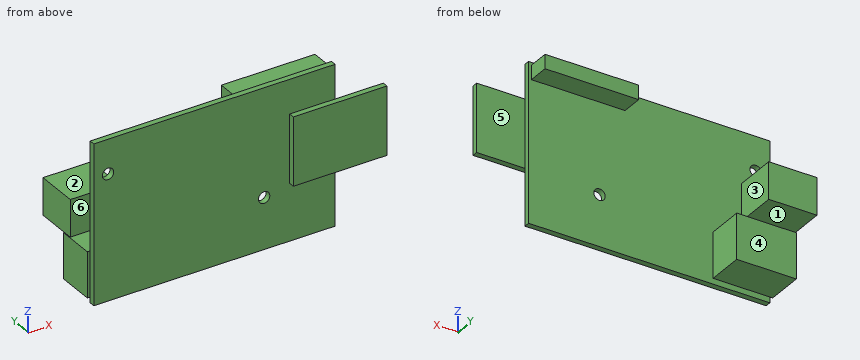
from build123d import *

# Parameters (mm, degrees)
SKETCH1_W           = 85
SKETCH1_H           = 56
BOSS_EXTRUDE1_DEPTH = 2
SKETCH2_W           = 21
SKETCH2_H           = 16
BOSS_EXTRUDE2_DEPTH = 13
SKETCH3_W           = 17
SKETCH3_H           = 13
BOSS_EXTRUDE3_DEPTH = 15
SKETCH4_W           = 33
SKETCH4_H           = 24
BOSS_EXTRUDE4_DEPTH = 2
CUT_EXTRUDE1_REACH  = 6
SKETCH5_R           = 2
SKETCH6_W           = 33
SKETCH6_H           = 5
BOSS_EXTRUDE5_DEPTH = 7.5


with BuildPart() as part:
    # Sketch1 → Boss-Extrude1 (new body)
    with BuildSketch(Plane(origin=(0, 0, 0), x_dir=(1, 0, 0), z_dir=(0, 1, 0))):
        with Locations((42.5, 28)):
            Rectangle(SKETCH1_W, SKETCH1_H)
    extrude(amount=BOSS_EXTRUDE1_DEPTH)

    # Sketch2 → Boss-Extrude2 (add)
    with BuildSketch(Plane(origin=(0, 2, 0), x_dir=(1, 0, 0), z_dir=(0, 1, 0))):
        with Locations((9.5, 46)):
            Rectangle(SKETCH2_W, SKETCH2_H)
    extrude(amount=BOSS_EXTRUDE2_DEPTH)

    # Sketch3 → Boss-Extrude3 (add)
    with BuildSketch(Plane(origin=(0, 2, 0), x_dir=(1, 0, 0), z_dir=(0, 1, 0))):
        with Locations((1.5, 24.5)):
            Rectangle(SKETCH3_W, SKETCH3_H)
    extrude(amount=BOSS_EXTRUDE3_DEPTH)

    # Sketch4 → Boss-Extrude4 (add)
    with BuildSketch(Plane.XZ):
        with Locations((85.5, -24)):
            Rectangle(SKETCH4_W, SKETCH4_H)
    extrude(amount=BOSS_EXTRUDE4_DEPTH)

    # Sketch5 → Cut-Extrude1 (cut, up to next)
    with BuildSketch(Plane(origin=(0, 2, 0), x_dir=(1, 0, 0), z_dir=(0, 1, 0)), mode=Mode.PRIVATE) as cut_extrude1_sk1:
        with Locations((5, 12)):
            Circle(SKETCH5_R)
    cut_extrude1_tool1 = extrude(cut_extrude1_sk1.sketch, amount=-CUT_EXTRUDE1_REACH, mode=Mode.PRIVATE) & part.part
    add(cut_extrude1_tool1.solids().sort_by_distance((5, 2, -12))[0], mode=Mode.SUBTRACT)
    # Sketch5 → Cut-Extrude1 (cut, up to next)
    with BuildSketch(Plane(origin=(0, 2, 0), x_dir=(1, 0, 0), z_dir=(0, 1, 0)), mode=Mode.PRIVATE) as cut_extrude1_sk2:
        with Locations((60, 38)):
            Circle(SKETCH5_R)
    cut_extrude1_tool2 = extrude(cut_extrude1_sk2.sketch, amount=-CUT_EXTRUDE1_REACH, mode=Mode.PRIVATE) & part.part
    add(cut_extrude1_tool2.solids().sort_by_distance((60, 2, -38))[0], mode=Mode.SUBTRACT)

    # Sketch6 → Boss-Extrude5 (add)
    with BuildSketch(Plane(origin=(0, 2, 0), x_dir=(1, 0, 0), z_dir=(0, 1, 0))):
        with Locations((67.5, 3.5)):
            Rectangle(SKETCH6_W, SKETCH6_H)
    extrude(amount=BOSS_EXTRUDE5_DEPTH)


solid = part.part
For this review, take the finished solid that the model builds, in its own axes (mm). Face numbers are marked on the shaded views. A direction names the side the tool comes from. Coordinates: 2 decimals unless noted, no trailing zeros. Loops run counter-clockwise (first coordinate to the right, second up) from the corner with the lowest first, then second, coordinate; pieces in that order, holes last. Notation, with made-up numbers: (30.25, 61) -> (81.25, 61) arc R18 cw to (81.25, 87) -> close; hole circle Ø4 at (59.25, 80). An arc over 180 degrees is marked (long way). Write each question's results on one line, items separated by ' | '.
Q1. Add section A-A, the plane y = 7.5. State the section outline as (x, z) points, then the cut area to 3 significant figures.
Taken from the geometry:
outline: (-7, -31) -> (10, -31) -> (10, -18) -> (-7, -18) -> close; (-1, -54) -> (20, -54) -> (20, -38) -> (-1, -38) -> close; (51, -6) -> (84, -6) -> (84, -1) -> (51, -1) -> close | area: 722 mm²
Q2. Mouldability with a two-part tool opening along Z and no side actions: class the marked faces 1, 2 and 3 as +Z half, -Z half, draft (parallel to the pull), parting line (faces both ways), or undercut.
Taken from the geometry:
face 1: undercut | face 2: +Z half | face 3: draft
Q3. To check wall thickness, follow line 1 along X through (y, z) = (0.8, -38); line 2 along X through (y, z) = (1.4, -12); line 3 along Z through (x, y) = (5, 0.45). State the ranges of each line that lie inside material, in increasing order. Write a range as [from, to].
Taken from the geometry:
line 1: [0, 58], [62, 85] | line 2: [0, 3], [7, 85] | line 3: [-56, -14], [-10, 0]
Q4. Add section C-C, the plane z = -4. State the section outline as (x, y) points, then the cut area to 4 significant figures.
Taken from the geometry:
outline: (0, 0) -> (85, 0) -> (85, 2) -> (84, 2) -> (84, 9.5) -> (51, 9.5) -> (51, 2) -> (0, 2) -> close | area: 417.5 mm²
Q5. For pin 1 Ø6.5 at (y, z) = (8, -26) entering from +X; pin 2 Ø10 at (y, z) = (6, -17.5) entering from +X; pin 3 Ø1.5 at (y, z) = (5.5, -3.5) entering from +X; pin 4 Ø1.5 at (y, z) = (11, -36) entering from -X, all flat-tipped, find the tip position at first contact; note any pin that passes through.
Taken from the geometry:
pin 1: x = 10 | pin 2: x = 85 | pin 3: x = 84 | pin 4: through
Q6. Add section B-B, the plane x = 60. State the section outline as (y, z) points, then the cut area to 4 significant figures.
Taken from the geometry:
outline: (0, -56) -> (2, -56) -> (2, -40) -> (0, -40) -> close; (0, -36) -> (2, -36) -> (2, -6) -> (9.5, -6) -> (9.5, -1) -> (2, -1) -> (2, 0) -> (0, 0) -> close | area: 141.5 mm²
Q7. Machinability: for the marked faces 4, 5 and 6, which of the approach directions +Z, -Z, +X, -X, +Y, -Y give a long, thin tool a straight path to every point of the face, cutting with its end or side? Answer none if there is none.
Taken from the geometry:
face 4: -Z, +X, -X, +Y | face 5: +Z, -Z, +X, +Y | face 6: +Z, -Z, -X, -Y
Q8. Add section D-D, the plane x = 1.5. State the section outline as (y, z) points, then the cut area to 3 significant figures.
Taken from the geometry:
outline: (0, -56) -> (2, -56) -> (2, -54) -> (15, -54) -> (15, -38) -> (2, -38) -> (2, -31) -> (17, -31) -> (17, -18) -> (2, -18) -> (2, 0) -> (0, 0) -> close | area: 515 mm²
